Verification items for the finished model (mm, model axes). Face numbers are marked on the shaded views. A direction names the side the tool comes from. Round coordinates to 2 decimals unless told otherwise and drop trailing zeros. Write each loop counter-clockwise with the first axis right and the second up, starting at its lowest first coordinate (ties: lowest second). Pieces come first, ordered by that corner, then holes.
Autodesk Inventor part; units mm, degrees
ref_plane "YZ Plane" through (0, 0, 0) normal (1, 0, 0) x (0, 1, 0)
ref_plane "XZ Plane" through (0, 0, 0) normal (0, 1, 0) x (-1, 0, 0)
ref_plane "XY Plane" through (0, 0, 0) normal (0, 0, 1) x (1, 0, 0)
sketch "Sketch1" plane through (0, 0, 0) normal (0, 0, 1) x (1, 0, 0)
  circle A0 centre (0, 0) radius 33.5
  circle A1 centre (0, 0) radius 33
  circle A2 centre (0, 0) radius 32.5
  dimension "d0" = 67
  dimension "d1" = 66
  dimension "d6" = 65
extrude "Extrusion1" add sketch "Sketch1" against normal blind 20 contours A0 | A1 | A2
extrude "Extrusion2" add sketch "Sketch1" along normal blind 15 contours A1 | A2
extrude "Extrusion3" add sketch "Sketch1" along normal blind 120 contours A2
chamfer "Chamfer1" distance 10 angle 45 1 edges at (-33.5, 0, -20)
chamfer "Chamfer2" [suppressed]
sketch "Sketch2" plane through (0, 0, -20) normal (0, 0, -1) x (-1, 0, 0)
  circle A0 centre (0, 0) radius 23.5
  line L0 (-12.5, 19.8997) -> (-12.5, -19.8997)
  line L1 (12.5, 19.8997) -> (12.5, -19.8997)
  dimension "d15" = 25
extrude "Extrusion4" add sketch "Sketch2" along normal blind 50 contours L1 A0 L0
sketch "Sketch3" plane through (12.5, -19.8997, -20) normal (1, 0, 0) x (0, 0, -1)
  line L0 (50, 39.7995) -> (50, 43.3997) construction
  line L1 (50, -3.6003) -> (50, 0) construction
  arc A0 (38.6481, -3.6003) -> (38.6481, 43.3997) centre (20, 19.8997) ccw
  line L2 (38.6481, 43.3997) -> (38.6481, -3.6003) construction
  line L3 (38.6481, 43.3997) -> (85.6481, 43.3997) construction
  line L4 (38.6481, 43.3997) -> (55.8157, 43.3997)
  line L5 (38.6481, -3.6003) -> (55.8157, -3.6003)
  line L6 (50, 39.7995) -> (50, 0) construction
  line L7 (55.8157, -3.6003) -> (55.8157, 43.3997)
  point P0 (-20, 19.8997)
  point P1 (62.1481, 43.3997)
  dimension "d19" = 90
  dimension "d48" = 30
extrude "Extrusion5" cut sketch "Sketch3" against normal through all
hole "Hole1" at (12.5, 0, -45) direction (-1, 0, 0) diameter 26 end through all
chamfer "Chamfer3" distance 2 angle 45 2 edges at (12.5, 0, -20) (-12.5, 0, -20)
hole "Hole2" at (0, 0, 120) direction (0, 0, -1) diameter 55 depth 120
chamfer "Chamfer4" distance 3 angle 45 1 edges at (-32.5, 0, 120)
chamfer "Chamfer5" distance 1 angle 45 2 edges at (-12.5, 0, -70) (12.5, 0, -70)
chamfer "Chamfer6" distance 2 angle 45 2 edges at (12.5, 0, -32) (-12.5, 0, -32)
properties part number "Base" material "Steel"
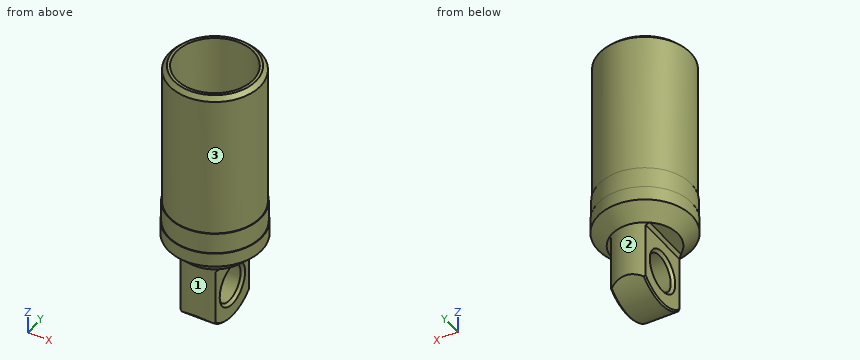
Q1. Sectioned sample at C-C (z = 54). Enter the section's corners in (x, y), plus the area to 3 significant figures.
Recorded:
outline: circle Ø65 at (0, 0); hole circle Ø55 at (0, 0)
area: 942 mm2
Q2. Sectioned sample at D-D (z = -6.5). Enter the section's corners in (x, y), plus the area to 3 significant figures.
Recorded:
outline: circle Ø67 at (0, 0)
area: 3,530 mm2
Q3. Depth check by flat-ended pin: P1, Ø12, axis at y = -15.5, z = 53.5, coming from the -X side; P2, Ø2, axis at x = 12, z = 17.5, coming from the +Y side; P3, Ø5, axis at y = 25, z = 18, coming from the -X side. Enter the tip coordinate at first touch or a pass-through.
Recorded:
P1: stops at x = -31.08
P2: stops at y = 30.58
P3: stops at x = -23.45
Q4. Sectioned sample at A-A (x = 0). Enter the section's corners in (y, z).
Recorded:
outline: (-33.5, -10) - (-23.5, -20) - (-23.5, -58.65) arc R30 ccw to (23.5, -58.65) - (23.5, -20) - (33.5, -10) - (33.5, 0) - (33, 0) - (33, 15) - (32.5, 15) - (32.5, 117) - (29.5, 120) - (27.5, 120) - (27.5, 0) - (-27.5, 0) - (-27.5, 120) - (-29.5, 120) - (-32.5, 117) - (-32.5, 15) - (-33, 15) - (-33, 0) - (-33.5, 0) - close; hole circle Ø26 at (0, -45)
Q5. Material ranges on line 1 along X through (y, z) = (0, 77); line 2 along Z through (x, y) = (1, 0); line 3 along Z through (x, y) = (14, 16), recorded low to high.
Recorded:
line 1: x = -32.5 to -27.5, 27.5 to 32.5
line 2: z = -70 to -58, -32 to 0
line 3: z = -20.5 to 0
Q6. Sectioned sample at B-B (z = -45). Enter the section's corners in (x, y), plus the area to 3 significant figures.
Recorded:
outline: (-12.5, -19.9) arc R23.5 ccw to (12.5, -19.9) - (12.5, -15) - (10.5, -13) - (-10.5, -13) - (-12.5, -15) - close; (-12.5, 15) - (-10.5, 13) - (10.5, 13) - (12.5, 15) - (12.5, 19.9) arc R23.5 ccw to (-12.5, 19.9) - close
area: 459 mm2
Q7. Tool access check on the marked faces 1, 2 and 3. Record the directions out of +Z, -Z, +X, -X, +Y, -Y that give a thin tool (end or side, any length) a straight path to the whole face; none if there is none.
Recorded:
face 1: -Z, -Y
face 2: -Z, +Y
face 3: +Z
